from build123d import *

# Parameters (mm, degrees)
F1_DEPTH = 7.5
F5_D     = 6.8


with BuildPart() as f1:
    # F0 (on Front) → F1 (new body)
    with BuildSketch(Plane.XZ):
        Polygon((6.5, -3.7527767497), (6.5, 3.7527767497), (0, 7.5055534995), (-6.5, 3.7527767497), (-6.5, -3.7527767497), (0, -7.5055534995), align=None)
    extrude(amount=-F1_DEPTH)

    # F2 (on Right) → F3 (revolve, cut)
    with BuildSketch(Plane.YZ):
        Polygon((0, 11.5055534995), (0, 6.5), (2.8899576604, 11.5055534995), align=None)
    revolve(axis=Axis((0, 2.7997596189, 0), (0, 1, 0)), mode=Mode.SUBTRACT)

    # F5 (through all)
    with Locations(Plane.XZ):
        with Locations((0, 0)):
            Hole(F5_D / 2)


solid = f1.part
Check sheet for the modelled part. Datum: model origin and axes. Units: mm. Round coordinates to 2 decimals unless told otherwise and drop trailing zeros. Order: outer loops, then holes, each group sorted by start corner. A loop starts at its lowest first (then second) coordinate and runs counter-clockwise, first axis right, second up.
Q1. Draft check along Z on faces 1 (the face through (-5.83, 0.14, -3.39)), 2 (the face through (3.3, 3.7, 5.6)), 3 (the face through (-2, 7.5, -3)), 4 (the face through (0.74, 3.8, -3.32)). Enter one of: pulls with the +Z half, pulls with the -Z half, needs draft (parallel to the pull), parting line crosses it, or undercut.
Filled sheet:
face 1: pulls with the -Z half
face 2: pulls with the +Z half
face 3: needs draft
face 4: undercut
Q2. Scan lines: L1, parallel to Z at x = 1.75, y = 6.5; L2, parallel to X at y = 3.5, z = 2.5; L3, parallel to Z at x = 3, y = 4.75. Record each from-to range of solid material in increasing order.
Filled sheet:
L1: z = -6.5 to -2.92, 2.92 to 6.5
L2: x = -6.5 to -2.3, 2.3 to 6.5
L3: z = -5.77 to -1.6, 1.6 to 5.77
Q3. Cross-section at A-A, the plane y = 2.25. Enter the section's corners in (x, z).
Filled sheet:
outline: (-6.5, -3.75) - (0, -7.51) - (6.5, -3.75) - (6.5, 3.75) - (0, 7.51) - (-6.5, 3.75) - close; hole circle Ø6.8 at (0, 0)
Q4. Depth check by flat-ended pin: P1, Ø6, axis at x = 0.5, z = 4.5, coming from the -Y side; P2, Ø2, axis at x = 2, y = 2, coming from the -Z side. Enter the tip coordinate at first touch or a pass-through.
Filled sheet:
P1: stops at y = 0
P2: stops at z = -6.93
